For this review, take the finished solid that the model builds, in its own axes (mm). A direction names the side the tool comes from. Give positions to 0.01 mm unless a question says otherwise; leave off trailing zeros. Order: outer loops, then holes, each group sorted by start corner. A loop starts at its lowest first (then second) coordinate and runs counter-clockwise, first axis right, second up. Notation, with made-up numbers: (31.25, -36) - (42.25, -36) arc R25 ccw to (42.25, -14) - close; hole circle Ø1 at (45.5, -3.75). An arc over 180 degrees is marked (long way). Put each result on its own line as item: value. Start each with the question number.
```python
from build123d import *

# Parameters (mm, degrees)
F0_W      = 70
F0_H      = 70
F1_DEPTH  = 70
F2_T      = -3
F3_W      = 8.89
F3_H      = 2.41
F3_W_2    = 7.2
F4_DEPTH  = 2.54
F5_W      = 3
F5_H      = 64
F6_DEPTH  = 8
F7_R      = 2.05
F8_DEPTH  = 3.302
F9_W      = 4.5
F9_H      = 48.4
F10_DEPTH = 99.568
F11_W     = 67
F11_H     = 2
F12_DEPTH = 1
F12_TAPER = -30
F14_DEPTH = 0.8
F16_DEPTH = 0.8
F17_W     = 7.2
F17_H     = 1.2938163138
F17_H_2   = 4.2561836862
F17_H_3   = 6.35
F18_DEPTH = 0.8
F20_DEPTH = 0.8
F21_W     = 3
F21_H     = 64
F22_DEPTH = 4.6


# Not quite as in the source:
# - a feature names something its author has since deleted; it is built from what else it names


with BuildPart() as f1:
    # F0 (on Top) → F1 (new body)
    with BuildSketch(Plane.XY):
        with Locations((1.2258447155, 1.6609302163)):
            Rectangle(F0_W, F0_H)
    extrude(amount=F1_DEPTH)

    # F2
    f2_openings = [f1.faces().sort_by_distance(p)[0] for p in [
        (36.225845, 1.66093, 35),
    ]]
    offset(amount=F2_T, openings=f2_openings)

    # F3 (on face) → F4 (cut)
    with BuildSketch(Plane.XY.offset(70)):
        with Locations((-4.6741552845, -4.6890697837)):
            Rectangle(F3_W, F3_H)
        with BuildLine():
            ThreePointArc((7.2258447155, -1.0290697837), (9.1279619569, -0.2411870251), (9.9158447155, 1.6609302163))
            ThreePointArc((9.9158447155, 1.6609302163), (9.1279619569, 3.5630474577), (7.2258447155, 4.3509302163))
            ThreePointArc((7.2258447155, 4.3509302163), (4.5358447155, 1.6609302163), (7.2258447155, -1.0290697837))
        make_face()
        with BuildLine():
            Line((9.9158447155, -1.0290697837), (9.9158447155, 1.6609302163))
            ThreePointArc((9.9158447155, 1.6609302163), (9.1279619569, -0.2411870251), (7.2258447155, -1.0290697837))
            Line((7.2258447155, -1.0290697837), (9.9158447155, -1.0290697837))
        make_face()
        with Locations((-4.6741552845, 8.0109302163)):
            Rectangle(F3_W_2, F3_H)
        with BuildLine():
            ThreePointArc((7.2258447155, 4.3509302163), (9.1279619569, 3.5630474577), (9.9158447155, 1.6609302163))
            Line((9.9158447155, 1.6609302163), (9.9158447155, 4.3509302163))
            Line((9.9158447155, 4.3509302163), (7.2258447155, 4.3509302163))
        make_face()
    extrude(amount=-F4_DEPTH, mode=Mode.SUBTRACT)

    # F5 (on face) → F6 (join)
    with BuildSketch(Plane(origin=(0, 0, 67), x_dir=(1, 0, 0), z_dir=(0, 0, -1))):
        with Locations((34.7258447155, -1.6609302163)):
            Rectangle(F5_W, F5_H)
    extrude(amount=F6_DEPTH)

    # F7 (on face) → F8 (cut)
    with BuildSketch(Plane(origin=(-33.7741552845, 0, 0), x_dir=(0, -1, 0), z_dir=(-1, 0, 0))):
        with Locations((-1.6609302163, 25.8598876931)):
            Circle(F7_R)
    extrude(amount=-F8_DEPTH, mode=Mode.SUBTRACT)

    # F9 (on face) → F10 (cut)
    with BuildSketch(Plane.XZ.offset(33.3390697837)):
        with Locations((28.9758447155, 30)):
            Rectangle(F9_W, F9_H)
    extrude(amount=-F10_DEPTH, mode=Mode.SUBTRACT)

    # F11 (on face) → F12 (cut)
    with BuildSketch(Plane.XY.offset(3)):
        with Locations((2.7258447155, 1.6609302163)):
            Rectangle(F11_W, F11_H)
    extrude(amount=-F12_DEPTH, taper=F12_TAPER, mode=Mode.SUBTRACT)

    # F13 (on face) → F14 (cut)
    with BuildSketch(Plane(origin=(0, 0, 67), x_dir=(1, 0, 0), z_dir=(0, 0, -1))):
        Polygon((-30.7741552845, -0.0109302163), (-30.7741552845, -3.3109302163), (1.0258447155, -3.3109302163), (1.7764000655, -4.6109302163), (1.7764000655, -5.1109302163), (12.5788900655, -5.1109302163), (12.5788900655, -4.6109302163), (13.3294454154, -3.3109302163), (33.2258447155, -3.3109302163), (33.2258447155, -0.0109302163), (13.3294454154, -0.0109302163), (12.5788900655, 1.2890697837), (12.5788900655, 1.7890697837), (1.7764000655, 1.7890697837), (1.7764000655, 1.2890697837), (1.0258447155, -0.0109302163), align=None)
    extrude(amount=-F14_DEPTH, mode=Mode.SUBTRACT)

    # F15 (on face) → F16 (cut)
    with BuildSketch(Plane(origin=(0, 0, 67), x_dir=(1, 0, 0), z_dir=(0, 0, -1))):
        Polygon((-30.7741552845, 5.0452534699), (-30.7741552845, 4.2452534699), (-12.6326995774, 4.2452534699), (-9.1191552845, 3.0155129674), (-0.2291552845, 3.0155129674), (3.2843890084, 4.2452534699), (33.2258447155, 4.2452534699), (33.2258447155, 5.0452534699), (3.2843890084, 5.0452534699), (-0.2291552845, 6.2749939724), (-9.1191552845, 6.2749939724), (-12.6326995774, 5.0452534699), align=None)
    extrude(amount=-F16_DEPTH, mode=Mode.SUBTRACT)

    # F17 (on face) → F18 (cut)
    with BuildSketch(Plane(origin=(0, 0, 67), x_dir=(1, 0, 0), z_dir=(0, 0, -1))):
        with Locations((29.6258447155, 5.6921616268)):
            Rectangle(F17_W, F17_H)
        with Locations((29.6258447155, 2.1171616268)):
            Rectangle(F17_W, F17_H_2)
        with Locations((29.6258447155, -6.4859302163)):
            Rectangle(F17_W, F17_H_3)
    extrude(amount=-F18_DEPTH, mode=Mode.SUBTRACT)

    # F19 (on face) → F20 (cut)
    with BuildSketch(Plane(origin=(0, 0, 67), x_dir=(1, 0, 0), z_dir=(0, 0, -1))):
        Polygon((26.0258447155, -8.4106897138), (26.0258447155, -7.6106897138), (2.4393890084, -7.6106897138), (-1.0741552845, -6.3809492113), (-8.2741552845, -6.3809492113), (-11.7876995774, -7.6106897138), (-30.7741552845, -7.6106897138), (-30.7741552845, -8.4106897138), (-11.7876995774, -8.4106897138), (-8.2741552845, -9.6404302163), (-1.0741552845, -9.6404302163), (2.4393890084, -8.4106897138), align=None)
    extrude(amount=-F20_DEPTH, mode=Mode.SUBTRACT)

    # F21 (on face) → F22 (cut)
    with BuildSketch(Plane(origin=(0, 0, 0), x_dir=(1, 0, 0), z_dir=(0, 0, -1))):
        with Locations((34.7258447155, -1.6609302163)):
            Rectangle(F21_W, F21_H)
    extrude(amount=-F22_DEPTH, mode=Mode.SUBTRACT)


solid = f1.part
```
1. Tool access review of faces 1 (the face through (1, 18, 3)), 2 (the face through (9.916, 2, 69)), 3 (the face through (29, 35, 5.8)), 4 (the face through (-3, 5, 67)): name each direction out of +Z, -Z, +X, -X, +Y, -Y from which nothing blocks a thin tool from reaching the whole face with its end or side.
2. Clearance check with a flat-ended pin moving along its axis: pin 1 (10 mm diameter, centred on y = 28, z = 17, fed in from +X). State where the tip first meets the part, or that it passes through.
3. Add section B-B, the plane y = 30. Give the boundary of the cut face in (x, z).
4. Add section C-C, the plane z = 55.5. Give the boundary of the cut face in (x, y).
5. Add section A-A, the plane z = 41. Give the boundary of the cut face in (x, y).
6. The part is to be moulded in two halves that separate along Z. For faces 5 (the face through (-32.3, 2.11, 23.86)), 6 (the face through (36.226, 4, 61)), say which applies: released by +Z, released by -Z, zero draft, split by the parting line, or undercut.
7. Wall thickness on line 1 (Z direction, x = 21, y = 2.5); line 2 (Z direction, x = -25, y = -17); line 3 (Y direction, x = 21, z = 4): over which ranges is each line inside the solid? List them lowest first. Write a range as from..to.
Found:
1. face 1: +X
1. face 2: +Z
1. face 3: +Y, -Y
1. face 4: none
2. pin 1: stops at x = -30.77
3. outline: (-33.77, 0) - (33.23, 0) - (33.23, 3) - (-30.77, 3) - (-30.77, 67) - (33.23, 67) - (33.23, 59) - (36.23, 59) - (36.23, 70) - (-33.77, 70) - close
4. outline: (-33.77, -33.34) - (36.23, -33.34) - (36.23, -30.34) - (-30.77, -30.34) - (-30.77, 33.66) - (36.23, 33.66) - (36.23, 36.66) - (-33.77, 36.66) - close
5. outline: (-33.77, -33.34) - (26.73, -33.34) - (26.73, -30.34) - (-30.77, -30.34) - (-30.77, 33.66) - (26.73, 33.66) - (26.73, 36.66) - (-33.77, 36.66) - close; (31.23, -33.34) - (36.23, -33.34) - (36.23, -30.34) - (31.23, -30.34) - close; (31.23, 33.66) - (36.23, 33.66) - (36.23, 36.66) - (31.23, 36.66) - close
6. face 5: undercut
6. face 6: zero draft
7. line 1: z = 0..2, 67.8..70
7. line 2: z = 0..3, 67..70
7. line 3: y = -33.34..-30.34, 33.66..36.66
